CAD build for the part. Positions are in the model's coordinates, mm. Round coordinates to 2 decimals unless told otherwise and drop trailing zeros. Loops run counter-clockwise (first coordinate to the right, second up) from the corner with the lowest first, then second, coordinate; pieces in that order, holes last. Notation, with made-up numbers: M 28.5,17 L 51.5,17 A22 cw 51.5,43 Z; hole C 62.25,-22 d8. An arc over 180 degrees is marked long. Use a Markdown table: item, result. Add a question column.
(1) Band-saw the part on B-B, the plane y = 45.5. Write the cut outline in (x, z).
(2) Band-saw the part on C-C, the plane z = 0.85. Write the cut outline in (x, y), and give its area (3 significant figures).
(3) Band-saw the part on D-D, the plane x = -7. Write the cut outline in (y, z).
(4) Wall check: L1, parallel to X at y = 50.5, z = 0.25; L2, parallel to Y at x = -45, z = -0.65; L3, parallel to Z at x = -50.5, y = 48.5. Give the ranges that are in metal, low to high.
(5) Band-saw the part on A-A, the plane x = 45. Write the cut outline in (y, z), and give its area (4 significant figures).
(6) Flat gauge pins, fed straight in: P1, Ø1.5, axis at x = -51.5, z = -0.5, coming from the -Y side; P2, Ø0.9, axis at y = -61, z = 0.5, coming from the -X side; P3, Ø1, axis at x = 50, z = 0.5, coming from the +Y side. Where does each tip first touch, or does it go through?
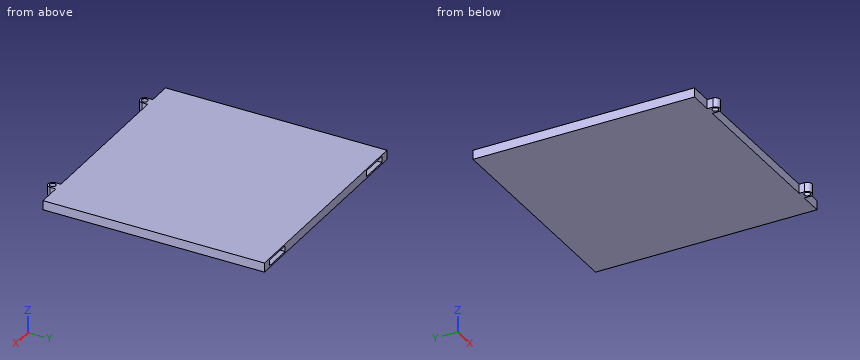
from build123d import *

# Parameters (mm, degrees)
SKETCH1_W           = 120
SKETCH1_H           = 120
BOSS_EXTRUDE1_DEPTH = 2.5
SKETCH4_W           = 15.2
SKETCH4_H           = 3.2
CUT_EXTRUDE1_DEPTH  = 20
SKETCH6_R           = 1.6
BOSS_EXTRUDE2_DEPTH = 5


with BuildPart() as part:
    # Sketch1 → Boss-Extrude1 (new, symmetric)
    with BuildSketch(Plane.XY):
        Rectangle(SKETCH1_W, SKETCH1_H)
    extrude(amount=BOSS_EXTRUDE1_DEPTH, both=True)

    # Sketch4 → Cut-Extrude1 (cut)
    with BuildSketch(Plane(origin=(0, 60, 0), x_dir=(1, 0, 0), z_dir=(0, 1, 0))):
        with Locations((-47.4, 0)):
            Rectangle(SKETCH4_W, SKETCH4_H)
        with Locations((47.4, 0)):
            Rectangle(SKETCH4_W, SKETCH4_H)
    extrude(amount=-CUT_EXTRUDE1_DEPTH, mode=Mode.SUBTRACT)

    # Sketch6 → Boss-Extrude2 (add)
    with BuildSketch(Plane.XY.offset(2.5)):
        with BuildLine():
            Line((42.5, -60), (47.5, -60))
            Line((47.5, -60), (47.5, -63))
            ThreePointArc((47.5, -63), (45, -65.5), (42.5, -63))
            Line((42.5, -63), (42.5, -60))
        make_face()
        with Locations((45, -63)):
            Circle(SKETCH6_R, mode=Mode.SUBTRACT)
    boss_extrude2 = extrude(amount=-BOSS_EXTRUDE2_DEPTH)

    # Mirror1: Boss-Extrude2 across plane
    add(boss_extrude2.mirror(Plane(origin=(0, 0, 0), x_dir=(0, 0, 1), z_dir=(1, 0, 0))))


solid = part.part
Return value:
| question | item | result |
|---|---|---|
| 1 | outline | M -60,-2.5 L 60,-2.5 L 60,2.5 L -60,2.5 Z; hole M -55,-1.6 L -39.8,-1.6 L -39.8,1.6 L -55,1.6 Z; hole M 39.8,-1.6 L 55,-1.6 L 55,1.6 L 39.8,1.6 Z |
| 2 | outline | M -60,-60 L -47.5,-60 L -47.5,-63 A2.5 ccw -42.5,-63 L -42.5,-60 L 42.5,-60 L 42.5,-63 A2.5 ccw 47.5,-63 L 47.5,-60 L 60,-60 L 60,60 L 55,60 L 55,40 L 39.8,40 L 39.8,60 L -39.8,60 L -39.8,40 L -55,40 L -55,60 L -60,60 Z; hole C -45,-63 d3.2; hole C 45,-63 d3.2 |
| 2 | area | 13,800 mm^2 |
| 3 | outline | M -60,-2.5 L 60,-2.5 L 60,2.5 L -60,2.5 Z |
| 4 | L1 | -60 to -55, -39.8 to 39.8, 55 to 60 |
| 4 | L2 | -65.5 to -64.6, -61.4 to 40 |
| 4 | L3 | -2.5 to -1.6, 1.6 to 2.5 |
| 5 | outline | M -65.5,-2.5 L -64.6,-2.5 L -64.6,2.5 L -65.5,2.5 Z; M -61.4,-2.5 L 60,-2.5 L 60,-1.6 L 40,-1.6 L 40,1.6 L 60,1.6 L 60,2.5 L -61.4,2.5 Z |
| 5 | area | 547.5 mm^2 |
| 6 | P1 | y = -60 |
| 6 | P2 | x = -47.5 |
| 6 | P3 | y = 40 |
